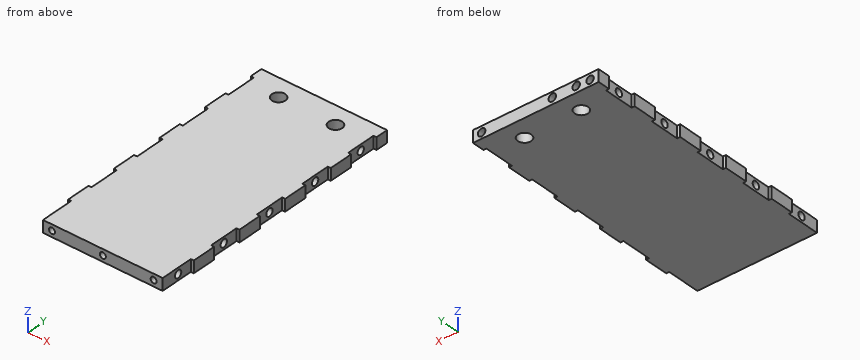
```python
from build123d import *

# Parameters (mm, degrees)
SKETCH_1_W              = 84
SKETCH_1_H              = 176.5
EXTRUDE_1_DEPTH         = 4
CUT_EXTRUDE1_DEPTH      = 99.061524055
CUT_EXTRUDE1_DEPTH_BACK = 99.061524055
SKETCH2_W               = 2
SKETCH2_H               = 20
SKETCH2_H_2             = 22.2
SKETCH2_W_2             = 86
SKETCH2_H_3             = 2
SKETCH3_R               = 2.5
CUT_EXTRUDE2_DEPTH      = 10
SKETCH4_R               = 2
CUT_EXTRUDE3_DEPTH      = 8
SKETCH5_R               = 2.5
CUT_EXTRUDE4_DEPTH      = 10
SKETCH6_R               = 4.5
CUT_EXTRUDE5_DEPTH      = 99.061524055
SKETCH7_R               = 2.5
CUT_EXTRUDE6_DEPTH      = 10


with BuildPart() as part:
    # 草图1 → 凸台-拉伸1 (new, symmetric)
    with BuildSketch(Plane.XY):
        Rectangle(SKETCH_1_W, SKETCH_1_H)
    extrude(amount=EXTRUDE_1_DEPTH, both=True)

    # Sketch2 → Cut-Extrude1 (cut, two sides: drawn at the far end of the back side and taken through both)
    with BuildSketch(Plane.XY.offset(4).offset(-CUT_EXTRUDE1_DEPTH_BACK)):
        with Locations((-41, 67.95)):
            Rectangle(SKETCH2_W, SKETCH2_H)
        with Locations((-41, 31.95)):
            Rectangle(SKETCH2_W, SKETCH2_H)
        with Locations((-41, -4.05)):
            Rectangle(SKETCH2_W, SKETCH2_H)
        with Locations((-41, -40.05)):
            Rectangle(SKETCH2_W, SKETCH2_H)
        with Locations((-41, -77.15)):
            Rectangle(SKETCH2_W, SKETCH2_H_2)
        with Locations((41, -77.15)):
            Rectangle(SKETCH2_W, SKETCH2_H_2)
        with Locations((41, -40.05)):
            Rectangle(SKETCH2_W, SKETCH2_H)
        with Locations((41, -4.05)):
            Rectangle(SKETCH2_W, SKETCH2_H)
        with Locations((41, 31.95)):
            Rectangle(SKETCH2_W, SKETCH2_H)
        with Locations((41, 67.95)):
            Rectangle(SKETCH2_W, SKETCH2_H)
        with Locations((0, 87.25)):
            Rectangle(SKETCH2_W_2, SKETCH2_H_3)
    extrude(amount=CUT_EXTRUDE1_DEPTH + CUT_EXTRUDE1_DEPTH_BACK, mode=Mode.SUBTRACT)

    # Sketch3 → Cut-Extrude2 (cut)
    with BuildSketch(Plane(origin=(40, 0, 0), x_dir=(0, 0, -1), z_dir=(1, 0, 0))):
        with Locations((0, 67.95)):
            Circle(SKETCH3_R)
        with Locations((0, 31.95)):
            Circle(SKETCH3_R)
        with Locations((0, -4.05)):
            Circle(SKETCH3_R)
        with Locations((0, -40.05)):
            Circle(SKETCH3_R)
        with Locations((0, -76.05)):
            Circle(SKETCH3_R)
    cut_extrude2 = extrude(amount=-CUT_EXTRUDE2_DEPTH, mode=Mode.SUBTRACT)

    # Mirror1: Cut-Extrude2 across plane
    add(cut_extrude2.mirror(Plane(origin=(0, 0, 0), x_dir=(0, 0, 1), z_dir=(1, 0, 0))), mode=Mode.SUBTRACT)

    # Sketch4 → Cut-Extrude3 (cut)
    with BuildSketch(Plane.XZ.offset(88.25)):
        with Locations(Location((-34, 0, 0), (0, 0, 270))):
            Circle(SKETCH4_R)
        with Locations(Location((34, 0, 0), (0, 0, 90))):
            Circle(SKETCH4_R)
        with Locations(Location((0, 0, 0), (0, 0, 270))):
            Circle(SKETCH4_R)
    extrude(amount=-CUT_EXTRUDE3_DEPTH, mode=Mode.SUBTRACT)

    # Sketch5 → Cut-Extrude4 (cut)
    with BuildSketch(Plane(origin=(0, 86.25, 0), x_dir=(1, 0, 0), z_dir=(0, 1, 0))):
        with Locations(Location((-36.25, 0, 0), (0, 0, 270))):
            Circle(SKETCH5_R)
        with Locations(Location((36.25, 0, 0), (0, 0, 270))):
            Circle(SKETCH5_R)
    extrude(amount=-CUT_EXTRUDE4_DEPTH, mode=Mode.SUBTRACT)

    # Sketch6 → Cut-Extrude5 (cut, through all)
    with BuildSketch(Plane(origin=(0, 0, -4), x_dir=(-1, 0, 0), z_dir=(0, 0, -1))):
        with Locations((-19, 72.75)):
            Circle(SKETCH6_R)
        with Locations(Location((19, 72.75, 0), (0, 0, 180))):
            Circle(SKETCH6_R)
    extrude(amount=-CUT_EXTRUDE5_DEPTH, mode=Mode.SUBTRACT)

    # Sketch7 → Cut-Extrude6 (cut)
    with BuildSketch(Plane(origin=(0, 86.25, 0), x_dir=(1, 0, 0), z_dir=(0, 1, 0))):
        with Locations(Location((-11, -0.32, 0), (0, 0, 270))):
            Circle(SKETCH7_R)
        with Locations(Location((-27, -0.32, 0), (0, 0, 270))):
            Circle(SKETCH7_R)
    extrude(amount=-CUT_EXTRUDE6_DEPTH, mode=Mode.SUBTRACT)


solid = part.part
```
For this review, take the finished solid that the model builds, in its own axes (mm). Round coordinates to 2 decimals unless told otherwise and drop trailing zeros. Write each loop counter-clockwise with the first axis right and the second up, starting at its lowest first coordinate (ties: lowest second). Pieces come first, ordered by that corner, then holes. Notation, with made-up numbers: (57.25, -39) - (77.25, -39) arc R26 ccw to (77.25, -8) - close; hole circle Ø9 at (30, 39). An arc over 180 degrees is marked (long way). Write each question's results on one line, items separated by ' | '.
Item 1: Take a section at B-B on y = 31.95. State the section outline as (x, z) points.
Calculated:
outline: (-40, -4) - (40, -4) - (40, -2.5) - (30, -2.5) - (30, 2.5) - (40, 2.5) - (40, 4) - (-40, 4) - (-40, 2.5) - (-30, 2.5) - (-30, -2.5) - (-40, -2.5) - close
Item 2: Take a section at D-D on x = 20. State the section outline as (y, z) points.
Calculated:
outline: (-88.25, -4) - (68.36, -4) - (68.36, 4) - (-88.25, 4) - close; (77.14, -4) - (86.25, -4) - (86.25, 4) - (77.14, 4) - close
Item 3: To check wall thickness, follow line 1 along Y through (x, z) = (-35.25, 0); line 2 along X through (y, z) = (-82.5, 0); line 3 along X through (y, z) = (83.75, 0). State the ranges of each line that lie inside material, in increasing order. Write a range as from..to.
Calculated:
line 1: y = -80.25..-78.55, -73.55..-42.55, -37.55..-6.55, -1.55..29.45, 34.45..65.45, 70.45..76.25 | line 2: x = -40..-36, -32..-2, 2..32, 36..40 | line 3: x = -42..-38.75, -33.75..-29.48, -24.52..-13.48, -8.52..33.75, 38.75..42
Item 4: Take a section at C-C on z = -0.75. Count the separate pieces of the cut face and the enclosed holes in it, then the cut area to 3 significant figures.
Calculated:
separate pieces: 1 | enclosed holes: 2 | area: 13,400 mm^2
Item 5: For pin 1 (2.5 mm diameter, centred on x = 36, z = 1, fed in from +Y); pin 2 (0.6 mm diameter, centred on x = 40.5, z = 1, fed in from -Y); pin 3 (1.5 mm diameter, centred on y = -75.5, z = 0, fed in from +X), all flat-tipped, find the tip position at first contact; note any pin that passes through.
Calculated:
pin 1: stops at y = 76.25 | pin 2: stops at y = -66.05 | pin 3: stops at x = 30
Item 6: Take a section at A-A on x = -19. State the section outline as (y, z) points.
Calculated:
outline: (-88.25, -4) - (68.25, -4) - (68.25, 4) - (-88.25, 4) - close; (77.25, -4) - (86.25, -4) - (86.25, 4) - (77.25, 4) - close
